```python
from build123d import *

# Parameters (mm, degrees)
SKETCH1_R           = 3
BOSS_EXTRUDE1_DEPTH = 5
BOSS_EXTRUDE2_START = 5
SKETCH1_3_R         = 4
SKETCH1_3_R_2       = 3
BOSS_EXTRUDE2_DEPTH = 1
BOSS_EXTRUDE3_START = -2
SKETCH1_4_R         = 6
SKETCH1_4_R_2       = 4
SKETCH1_4_R_3       = 3
BOSS_EXTRUDE3_DEPTH = 2
CHAMFER1_SIZE       = 0.5


with BuildPart() as part:
    # Sketch1 → Boss-Extrude1 (new body)
    with BuildSketch(Plane.XY):
        Circle(SKETCH1_R)
    extrude(amount=BOSS_EXTRUDE1_DEPTH)

    # Sketch1<3> → Boss-Extrude2 (add)
    # profile 1 of 2: a face of its own
    with BuildSketch(Plane.XY.offset(BOSS_EXTRUDE2_START)):
        Circle(SKETCH1_3_R)
        Circle(SKETCH1_3_R_2, mode=Mode.SUBTRACT)
    # profile 2 of 2: a face of its own
    with BuildSketch(Plane.XY.offset(BOSS_EXTRUDE2_START)):
        Circle(SKETCH1_3_R_2)
    extrude(amount=BOSS_EXTRUDE2_DEPTH)

    # Sketch1<4> → Boss-Extrude3 (add)
    # profile 1 of 3: a face of its own
    with BuildSketch(Plane.XY.offset(BOSS_EXTRUDE3_START)):
        Circle(SKETCH1_4_R)
        Circle(SKETCH1_4_R_2, mode=Mode.SUBTRACT)
    # profile 2 of 3: a face of its own
    with BuildSketch(Plane.XY.offset(BOSS_EXTRUDE3_START)):
        Circle(SKETCH1_4_R_2)
        Circle(SKETCH1_4_R_3, mode=Mode.SUBTRACT)
    # profile 3 of 3: a face of its own
    with BuildSketch(Plane.XY.offset(BOSS_EXTRUDE3_START)):
        Circle(SKETCH1_4_R_3)
    extrude(amount=BOSS_EXTRUDE3_DEPTH)

    # Chamfer1
    chamfer1_edges = [part.edges().sort_by_distance(p)[0] for p in [
        (-6, 0, -2),
    ]]
    chamfer(chamfer1_edges, length=CHAMFER1_SIZE)


solid = part.part
```
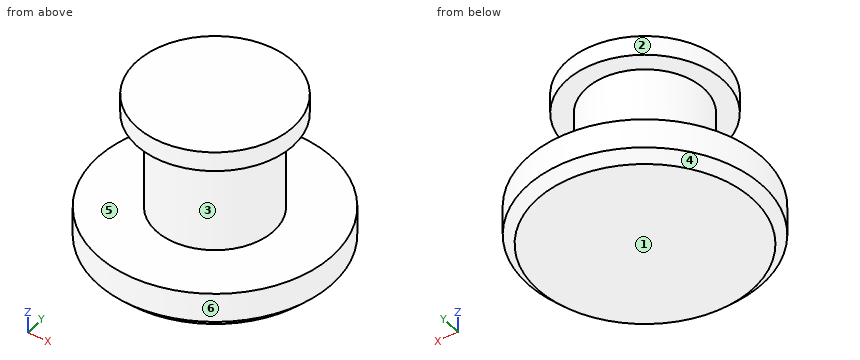
Source: CAD feature listing. Evaluate the final solid. Frame: model axes, mm. Face numbers are marked on the shaded views. A direction names the side the tool comes from. Round coordinates to 2 decimals unless told otherwise and drop trailing zeros. Loops run counter-clockwise (first coordinate to the right, second up) from the corner with the lowest first, then second, coordinate; pieces in that order, holes last.
(1) Contact query for flat-ended pins moving along their axis: pin 1 Ø3 at (y, z) = (3, -1) entering from +X; pin 2 Ø4 at (y, z) = (-4, 1) entering from +X; pin 3 Ø2 at (x, z) = (-2.5, 2.5) entering from -Y. Output: stop coordinate, or through.
From the geometry:
pin 1: stops at x = 5.81
pin 2: stops at x = 5.55
pin 3: stops at y = -2.6
(2) Section query A-A (x = 0). Output: boundary loops of the cut face in (y, z).
From the geometry:
outline: (-6, -1.5) - (-5.5, -2) - (5.5, -2) - (6, -1.5) - (6, 0) - (3, 0) - (3, 5) - (4, 5) - (4, 6) - (-4, 6) - (-4, 5) - (-3, 5) - (-3, 0) - (-6, 0) - close
(3) Pull-direction query (Z, two-part tool) for the marked faces 4, 5 and 6; classes: +Z half, -Z half, draft (parallel to the pull), parting line (faces both ways), or undercut.
From the geometry:
face 4: -Z half
face 5: undercut
face 6: draft
(4) Access query for the marked faces 1, 2 and 3. Directions: +Z, -Z, +X, -X, +Y, -Y. A direction counts if a zero-diameter tool reaches every point of the face in a straight line with its end or side. Return the directions, or none.
From the geometry:
face 1: -Z, +X, -X, +Y, -Y
face 2: +Z
face 3: none
(5) Section query C-C (z = 3.5). Output: boundary loops of the cut face in (x, y), and give its area (3 significant figures).
From the geometry:
outline: circle Ø6 at (0, 0)
area: 28.3 mm2
(6) Material intervals for probe 1 along Z at (x, y) = (-3, -2); probe 2 along Z at (x, y) = (-3.75, -3); probe 3 along Y at (x, z) = (4.5, -1), sorted ascending.
From the geometry:
probe 1: z = -2 to 0, 5 to 6
probe 2: z = -2 to 0
probe 3: y = -3.97 to 3.97
